For this review, take the finished solid that the model builds, in its own axes (mm). A direction names the side the tool comes from. Round coordinates to 2 decimals unless told otherwise and drop trailing zeros. Order: outer loops, then holes, each group sorted by start corner. A loop starts at its lowest first (then second) coordinate and runs counter-clockwise, first axis right, second up. Notation, with made-up numbers: M 54.5,-29 L 61.5,-29 A18 cw 61.5,-16 Z; hole C -3.5,10 d7. An arc over 180 degrees is marked long. Write item = value, one per line. Start each with the question number.
from build123d import *

# Parameters (mm, degrees)
F0_R     = 19
F1_DEPTH = 24
F1_TAPER = -4
F2_R     = 8
F3_DEPTH = 24.0010001
F2_R_2   = 11
F4_DEPTH = 6
F5_R     = 11
F5_R_2   = 8
F6_DEPTH = 6


with BuildPart() as f1:
    # F0 (on Top) → F1 (new body)
    with BuildSketch(Plane.XY):
        Circle(F0_R)
    extrude(amount=F1_DEPTH, taper=F1_TAPER)

    # F2 (on face) → F3 (cut, through all)
    with BuildSketch(Plane(origin=(0, 0, 0), x_dir=(1, 0, 0), z_dir=(0, 0, -1))):
        Circle(F2_R)
    extrude(amount=-F3_DEPTH, mode=Mode.SUBTRACT)

    # F2 (on face) → F4 (cut)
    with BuildSketch(Plane(origin=(0, 0, 0), x_dir=(1, 0, 0), z_dir=(0, 0, -1))):
        Circle(F2_R_2)
        Circle(F2_R, mode=Mode.SUBTRACT)
    extrude(amount=-F4_DEPTH, mode=Mode.SUBTRACT)

    # F5 (on face) → F6 (cut)
    with BuildSketch(Plane.XY.offset(24)):
        Circle(F5_R)
        Circle(F5_R_2, mode=Mode.SUBTRACT)
    extrude(amount=-F6_DEPTH, mode=Mode.SUBTRACT)


solid = f1.part
(1) We need section A-A, the plane x = 0. Write out the cut boundary in (y, z), then the cut area to 3 significant figures.
(2) Draft analysis for pull direction Y (two halves, no side actions). For faces 1 (the cylindrical face through (-2.38, -10.74, 21.04)), 2 (the flat face through (9, -9, 24)), 3 (the conical face through (-15.6, -11.97, 9.5)), 4 (the flat face through (-2, 8, 6)), state which applies: released by +Y, released by -Y, zero draft, split by the parting line, or undercut.
(3) We need section C-C, the plane z = 7. Write out the cut boundary in (x, y).
(4) We need section B-B, the plane z = 2.5. Write out the cut boundary in (x, y).
(5) Insertion check: pin 1 (10 mm diameter, centred on y = 4.5, z = 7.5, fed in from +X); pin 2 (4 mm diameter, centred on x = 16.5, z = 9.5, fed in from -Y); pin 3 (11 mm diameter, centred on x = 0, y = 3, fed in from +Z); pin 4 (11 mm diameter, centred on x = -1, y = 1.5, fed in from -Z). Each pin has a flat end and moves straight along its axis. Give the tip position at first contact, or say it passes through.
(6) For line 1 along Y through (x, z) = (0, 22.75); line 2 along X through (y, z) = (2.5, 4.5); line 3 along Y through (x, z) = (2, 22), list the stretches that pass through material, from the lowest coordinate up.
(7) For faces 5 (the flat face through (8, -8, 0)), 6 (the cylindrical face through (-2.38, 10.74, 2.96)), 7 (the flat face through (-2, -8, 18)), list the 3-axis set-ups (+Z, -Z, +X, -X, +Y, -Y) from which the entire face can be reached by the end or side of a thin tool; tool diameter is ignored.
Values:
q1.outline = M -20.68,24 L -19,0 L -11,0 L -11,6 L -8,6 L -8,18 L -11,18 L -11,24 Z; M 8,6 L 11,6 L 11,0 L 19,0 L 20.68,24 L 11,24 L 11,18 L 8,18 Z
q1.area = 496 mm²
q2.face_1 = undercut
q2.face_2 = zero draft
q2.face_3 = split by the parting line
q2.face_4 = undercut
q3.outline = C 0,0 d38.98; hole C 0,0 d16
q4.outline = C 0,0 d38.35; hole C 0,0 d22
q5.pin_1 = 19.75
q5.pin_2 = -13.29
q5.pin_3 = 18
q5.pin_4 = through
q6.line_1 = -20.59 to -11, 11 to 20.59
q6.line_2 = -19.15 to -10.71, 10.71 to 19.15
q6.line_3 = -20.44 to -10.82, 10.82 to 20.44
q7.face_5 = -Z, +X, -X, +Y, -Y
q7.face_6 = -Z
q7.face_7 = +Z
